Design review of the part shown in the three views and the two pictorial views. Dimensions are in mm from the part's minimum x, y and z. A direction names the side the tool comes from. Round coordinates to 2 decimals unless told otherwise and drop trailing zeros. Write each loop counter-clockwise with the first axis right and the second up, starting at its lowest first coordinate (ties: lowest second). Pieces come first, ordered by that corner, then holes. Notation, with made-up numbers: (44.5, 74) - (77.5, 74) arc R16 cw to (77.5, 87) - close; hole circle Ø3 at (49.25, 45). An arc over 180 degrees is marked (long way). Use one line per item in the form item = value.
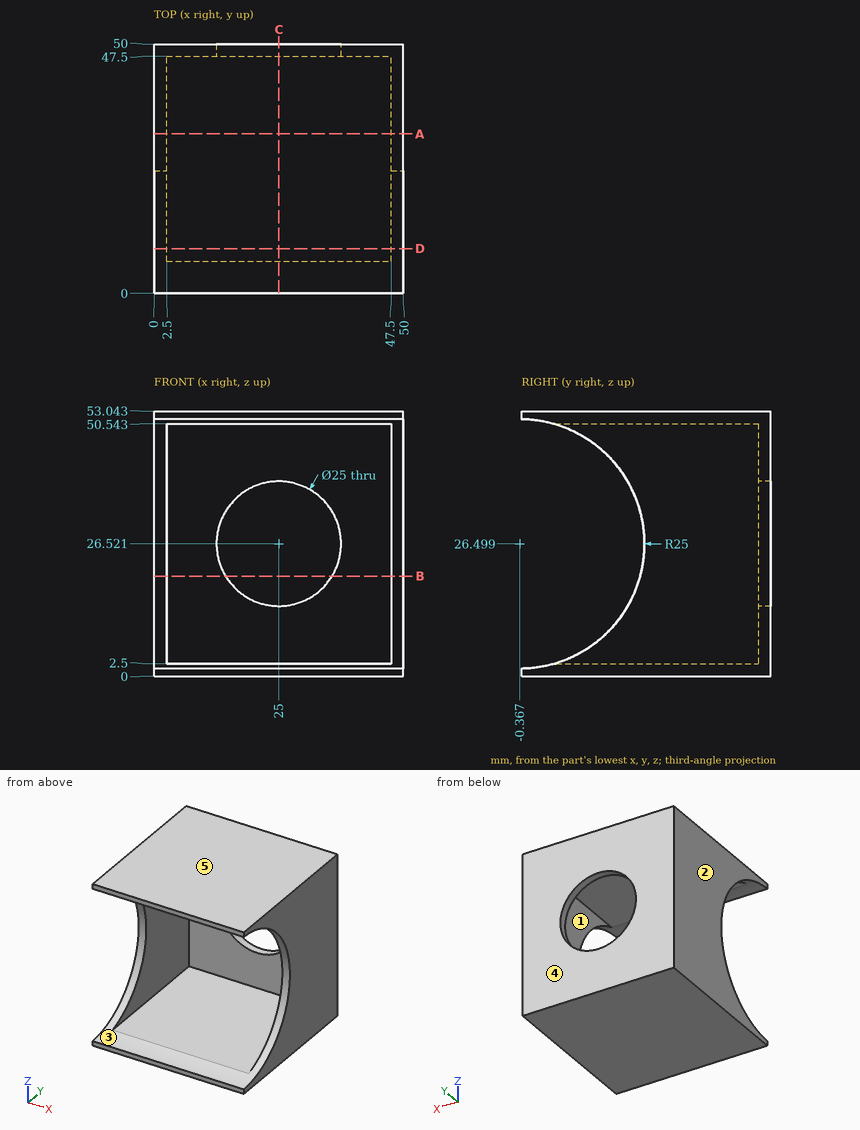
(1) Add section B-B on z = 20. Write out the cut boundary in (x, y).
Geometry results:
outline = (0, 23.77) - (2.5, 23.77) - (2.5, 47.5) - (14.34, 47.5) - (14.34, 50) - (0, 50) - close; (35.66, 47.5) - (47.5, 47.5) - (47.5, 23.77) - (50, 23.77) - (50, 50) - (35.66, 50) - close
(2) Add section C-C on x = 25. Write out the cut boundary in (y, z) (1 decimal).
Geometry results:
outline = (0, 0) - (50, 0) - (50, 14) - (47.5, 14) - (47.5, 2.5) - (6.6, 2.5) arc R25 cw to (0, 1.5) - close; (0, 51.5) arc R25 cw to (6.5, 50.5) - (47.5, 50.5) - (47.5, 39) - (50, 39) - (50, 53) - (0, 53) - close
(3) Machinability: for the marked faces 1 and 2, which of the approach directions +Z, -Z, +X, -X, +Y, -Y give a long, thin tool a straight path to every point of the face, cutting with its end or side? Answer none if there is none.
Geometry results:
face_1 = -Y
face_2 = +Z, -Z, -X, +Y, -Y
(4) The part is to be moulded in two halves that separate along Z. For the marked faces 3, 4 and 5, say which applies: +Z half, -Z half, draft (parallel to the pull), parting line (faces both ways), or undercut.
Geometry results:
face_3 = undercut
face_4 = draft
face_5 = +Z half
(5) Insertion check: P1, Ø1.5, axis at x = 12.5, z = 42, coming from the -Y side. The pin has a flat end and moves straight along its axis. Give the tip position at first contact, or say it passes through.
Geometry results:
P1 = 47.5
(6) Add section A-A on y = 32. Write out the cut boundary in (x, z).
Geometry results:
outline = (0, 0) - (50, 0) - (50, 53.04) - (0, 53.04) - close; hole (2.5, 2.5) - (47.5, 2.5) - (47.5, 50.54) - (2.5, 50.54) - close
(7) Add section D-D on y = 9. Write out the cut boundary in (x, z).
Geometry results:
outline = (0, 0) - (50, 0) - (50, 3.32) - (47.5, 3.32) - (47.5, 2.5) - (2.5, 2.5) - (2.5, 3.32) - (0, 3.32) - close; (0, 49.68) - (2.5, 49.68) - (2.5, 50.54) - (47.5, 50.54) - (47.5, 49.68) - (50, 49.68) - (50, 53.04) - (0, 53.04) - close
(8) To check wall thickness, follow L1, parallel to X at y = 46, z = 23.5; L2, parallel to Z at x = 42, y = 15.5; L3, parallel to Z at x = 25, y = 48. State the ranges of each line that lie inside material, in increasing order.
Geometry results:
L1 = 0 to 2.5, 47.5 to 50
L2 = 0 to 2.5, 50.54 to 53.04
L3 = 0 to 14.02, 39.02 to 53.04
